from build123d import *

# Parameters (mm, degrees)
SKETCH1_R           = 1.26
BOSS_EXTRUDE1_DEPTH = 3.5
FILLET1_R           = 1


with BuildPart() as part:
    # Sketch1 → Boss-Extrude1 (new body)
    # profile 1 of 2: a face of its own
    with BuildSketch(Plane.XY):
        with BuildLine():
            Line((3.5, 10.5), (0, 10.5))
            Line((0, 10.5), (0, 3.5))
            Line((0, 3.5), (8.5, 3.5))
            Line((8.5, 3.5), (8.5, 0))
            Line((8.5, 0), (23.5, 0))
            Line((23.5, 0), (23.5, 3.5))
            Line((23.5, 3.5), (26.7, 3.5))
            Line((26.7, 3.5), (26.7, 7.5))
            Line((26.7, 7.5), (35.7, 7.5))
            Line((35.7, 7.5), (35.7, 32.54836019))
            ThreePointArc((35.7, 32.54836019), (20.513860835, 22.69057725), (3.5, 16.5))
            Line((3.5, 16.5), (3.5, 10.5))
        make_face()
    # profile 2 of 2: a face of its own
    with BuildSketch(Plane.XY):
        with BuildLine():
            ThreePointArc((48.657927336, 46.063814965), (42.575731037, 38.925687301), (35.7, 32.54836019))
            Line((35.7, 32.54836019), (35.7, 7.5))
            Line((35.7, 7.5), (44.7, 7.5))
            Line((44.7, 7.5), (44.7, 3.5))
            Line((44.7, 3.5), (47.9, 3.5))
            Line((47.9, 3.5), (47.9, 0))
            Line((47.9, 0), (62.9, 0))
            Line((62.9, 0), (62.9, 3.5))
            Line((62.9, 3.5), (71.5, 3.5))
            Line((71.5, 3.5), (71.5, 12.5))
            Line((71.5, 12.5), (67.5, 12.5))
            Line((67.5, 12.5), (63.691186196, 42.073003524))
            ThreePointArc((63.691186196, 42.073003524), (57.515260243, 49.118796295), (48.657927336, 46.063814965))
        make_face()
        with Locations((55.75, 41.5)):
            Circle(SKETCH1_R, mode=Mode.SUBTRACT)
    extrude(amount=BOSS_EXTRUDE1_DEPTH)

    # Fillet1
    fillet1_edges = [part.edges().sort_by_distance(p)[0] for p in [
        (67.5, 12.5, 1.75),
    ]]
    fillet(fillet1_edges, radius=FILLET1_R)


solid = part.part
The model under review builds one solid part; all positions refer to its coordinate system, in mm. A direction names the side the tool comes from. Round coordinates to 2 decimals unless told otherwise and drop trailing zeros. Loops run counter-clockwise (first coordinate to the right, second up) from the corner with the lowest first, then second, coordinate; pieces in that order, holes last. Notation, with made-up numbers: (72.5, -34.5) -> (114.5, -34.5) arc R30 ccw to (114.5, -4.5) -> close; hole circle Ø7 at (-14.75, 1). An arc over 180 degrees is marked (long way). One line per question, with ' | ' between items. Start each with the question number.
Item 1: Add section D-D, the plane x = 25.5. Write out the cut boundary in (y, z), then the cut area to 3 significant figures.
Item 2: Draft analysis for pull direction X (two halves, no side actions). For faces 1 (the face through (36, 7.5, 2)), 2 (the face through (55, 0, 2)), 3 (the face through (62.9, 2, 2)), state which applies: +X half, -X half, draft (parallel to the pull), parting line (faces both ways), or undercut.
Item 3: Wall thickness on line 1 along X through (y, z) = (4, 1.6); line 2 along Y through (x, z) = (55.75, 1.35); line 3 along X through (y, z) = (2.5, 2.2): over which ranges is each line inside the solid? List them lowest first. Write a range as [from, to].
Item 4: Add section A-A, the plane x = 55.75. Write out the cut boundary in (y, z).
Item 5: Add section B-B, the plane z = 1.15. Write out the cut boundary in (x, y).
Item 6: For pin 1 (1 mm diameter, centred on y = 2, z = 2, fed in from -X); pin 2 (1 mm diameter, centred on x = 62, y = 33, fed in from -Z); pin 3 (2 mm diameter, centred on y = 24, z = 0.5, fed in from -X); pin 4 (1 mm diameter, centred on y = 28.5, z = 2, fed in from +X), all flat-tipped, find the tip position at first contact; note any pin that passes through.
Item 7: Machinability: for faces 4 (the face through (2, 10.5, 2)), 5 (the face through (4, 3.5, 2)), 6 (the face through (23.5, 2, 2)), which of the approach directions +Z, -Z, +X, -X, +Y, -Y give a long, thin tool a straight path to every point of the face, cutting with its end or side? Answer none if there is none.
Item 8: Add section C-C, the plane y = 11.5. Write out the cut boundary in (x, z).
Return value:
1) outline: (3.5, 0) -> (25.4, 0) -> (25.4, 3.5) -> (3.5, 3.5) -> close | area: 76.7 mm2
2) face 1: undercut | face 2: draft | face 3: +X half
3) line 1: x = [0, 26.7], [44.7, 71.5] | line 2: y = [0, 40.24], [42.76, 49.39] | line 3: x = [8.5, 23.5], [47.9, 62.9]
4) outline: (0, 0) -> (40.24, 0) -> (40.24, 3.5) -> (0, 3.5) -> close; (42.76, 0) -> (49.39, 0) -> (49.39, 3.5) -> (42.76, 3.5) -> close
5) outline: (0, 3.5) -> (8.5, 3.5) -> (8.5, 0) -> (23.5, 0) -> (23.5, 3.5) -> (26.7, 3.5) -> (26.7, 7.5) -> (44.7, 7.5) -> (44.7, 3.5) -> (47.9, 3.5) -> (47.9, 0) -> (62.9, 0) -> (62.9, 3.5) -> (71.5, 3.5) -> (71.5, 12.5) -> (68.38, 12.5) arc R1 cw to (67.39, 13.37) -> (63.69, 42.07) arc R8.4 ccw to (48.66, 46.06) arc R80 cw to (3.5, 16.5) -> (3.5, 10.5) -> (0, 10.5) -> close; hole circle Ø2.52 at (55.75, 41.5)
6) pin 1: stops at x = 8.5 | pin 2: stops at z = 0 | pin 3: stops at x = 21.13 | pin 4: stops at x = 65.5
7) face 4: +Z, -Z, -X, +Y | face 5: +Z, -Z, -X, -Y | face 6: +Z, -Z, -Y
8) outline: (3.5, 0) -> (71.5, 0) -> (71.5, 3.5) -> (3.5, 3.5) -> close
